Model file for the job. Use its own axes, mm. Face numbers are marked on the shaded views. Round coordinates to 2 decimals unless told otherwise and drop trailing zeros. Loops run counter-clockwise (first coordinate to the right, second up) from the corner with the lowest first, then second, coordinate; pieces in that order, holes last. Notation, with made-up numbers: (39, 70) - (86, 70) arc R20 cw to (86, 87) - close; hole circle Ø3 at (76, 89). An arc over 180 degrees is marked (long way). Answer as a JSON object with one key per item and string values.
from build123d import *

# Parameters (mm, degrees)
SKETCH1_W           = 177.8
SKETCH1_H           = 177.8
BOSS_EXTRUDE1_DEPTH = 6.35
SKETCH2_R           = 7.9375
CUT_EXTRUDE1_DEPTH  = 126.88384527
SKETCH3_W           = 96.606953724
SKETCH3_H           = 25.4
BOSS_EXTRUDE2_DEPTH = 38.1
CUT_EXTRUDE2_REACH  = 194.71
SKETCH4_W           = 71.206953724
SKETCH4_H           = 33.02
SKETCH5_R           = 6.35
CUT_EXTRUDE3_DEPTH  = 170.421977804


with BuildPart() as part:
    # Sketch1 → Boss-Extrude1 (new body)
    with BuildSketch(Plane(origin=(0, 0, 0), x_dir=(1, 0, 0), z_dir=(0, 1, 0))):
        Rectangle(SKETCH1_W, SKETCH1_H)
    extrude(amount=BOSS_EXTRUDE1_DEPTH)

    # Sketch2 → Cut-Extrude1 (cut, through all)
    with BuildSketch(Plane(origin=(0, 6.35, 0), x_dir=(1, 0, 0), z_dir=(0, 1, 0))):
        with Locations(Location((0, -12.7, 0), (0, 0, 270))):
            Circle(SKETCH2_R)
    extrude(amount=-CUT_EXTRUDE1_DEPTH, mode=Mode.SUBTRACT)

    # Sketch3 → Boss-Extrude2 (add)
    with BuildSketch(Plane(origin=(0, 6.35, 0), x_dir=(1, 0, 0), z_dir=(0, 1, 0))):
        with Locations((0, 63.5)):
            Rectangle(SKETCH3_W, SKETCH3_H)
    extrude(amount=BOSS_EXTRUDE2_DEPTH)

    # Sketch4 → Cut-Extrude2 (cut, up to next)
    with BuildSketch(Plane(origin=(0, 0, -76.2), x_dir=(-1, 0, 0), z_dir=(0, 0, -1)), mode=Mode.PRIVATE) as cut_extrude2_sk1:
        with Locations((0, 27.94)):
            Rectangle(SKETCH4_W, SKETCH4_H)
    cut_extrude2_tool1 = extrude(cut_extrude2_sk1.sketch, amount=-CUT_EXTRUDE2_REACH, mode=Mode.PRIVATE) & part.part
    add(cut_extrude2_tool1.solids().sort_by_distance((0, 27.94, -76.2))[0], mode=Mode.SUBTRACT)

    # Sketch5 → Cut-Extrude3 (cut, through all)
    with BuildSketch(Plane.ZY.offset(48.303476862)):
        with Locations((-63.5, 31.75)):
            Circle(SKETCH5_R)
    extrude(amount=-CUT_EXTRUDE3_DEPTH, mode=Mode.SUBTRACT)


solid = part.part
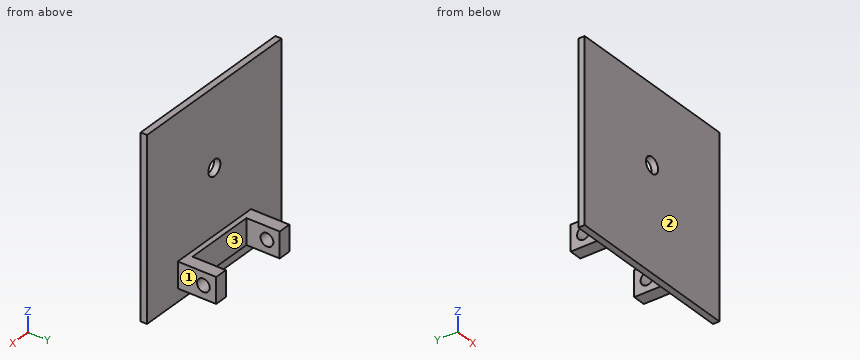
1) Probe probe 1 along Z at (x, y) = (40, 31); probe 2 along Y at (x, z) = (-41.5, -63.5); probe 3 along X at (y, z) = (40, -52). List the from-to ranges inside material, lowest first.
Values follow:
{"probe 1": "-76.2 to -69.81, -57.19 to -50.8", "probe 2": "0 to 25.4, 38.1 to 44.45", "probe 3": "-48.3 to -35.6, 35.6 to 48.3"}
2) Drop flat-ended pins along their axis: P1, Ø20.5, axis at y = 31.75, z = -63.5, coming from the +X side; P2, Ø12.5, axis at x = 14, z = -66.5, coming from the +Y side; P3, Ø12.5, axis at y = 27, z = -65.5, coming from the -X side. Give the stop position or say it passes through.
Values follow:
{"P1": "x = 48.3", "P2": "y = 11.43", "P3": "x = -48.3"}
3) Two-plate mould, pull along X, no slides. Class the marked faces 1, 2 and 3: pulls with the +X half, pulls with the -X half, needs draft (parallel to the pull), parting line crosses it, or undercut.
Values follow:
{"face 1": "pulls with the +X half", "face 2": "needs draft", "face 3": "undercut"}
4) Slice it at D-D on x = 43.5. List the corners of the cut face in (y, z), then the cut area to 3 significant figures.
Values follow:
{"outline": "(0, -88.9) - (6.35, -88.9) - (6.35, -76.2) - (44.45, -76.2) - (44.45, -50.8) - (6.35, -50.8) - (6.35, 88.9) - (0, 88.9) - close; hole circle Ø12.7 at (31.75, -63.5)", "area": "1,970 mm²"}
5) Slice it at C-C on x = 0. List the corners of the cut face in (y, z).
Values follow:
{"outline": "(0, -88.9) - (6.35, -88.9) - (6.35, -76.2) - (11.43, -76.2) - (11.43, -50.8) - (6.35, -50.8) - (6.35, 4.76) - (0, 4.76) - close; (0, 20.64) - (6.35, 20.64) - (6.35, 88.9) - (0, 88.9) - close"}
6) Slice it at A-A on y = 31.75. List the corners of the cut face in (x, z), then the cut area to 3 significant figures.
Values follow:
{"outline": "(-48.3, -76.2) - (-35.6, -76.2) - (-35.6, -69.85) - (-48.3, -69.85) - close; (-48.3, -57.15) - (-35.6, -57.15) - (-35.6, -50.8) - (-48.3, -50.8) - close; (35.6, -76.2) - (48.3, -76.2) - (48.3, -69.85) - (35.6, -69.85) - close; (35.6, -57.15) - (48.3, -57.15) - (48.3, -50.8) - (35.6, -50.8) - close", "area": "323 mm²"}
7) Slice it at B-B on z = 12.7. List the corners of the cut face in (x, y), then the cut area to 3 significant figures.
Values follow:
{"outline": "(-88.9, 0) - (-7.94, 0) - (-7.94, 6.35) - (-88.9, 6.35) - close; (7.94, 0) - (88.9, 0) - (88.9, 6.35) - (7.94, 6.35) - close", "area": "1,030 mm²"}
